Geometry: see drawing. Coordinates: mm, zero at the bounding-box minimum. A direction names the side the tool comes from. Coordinates: 2 decimals unless noted, no trailing zeros. Loops run counter-clockwise (first coordinate to the right, second up) from the corner with the lowest first, then second, coordinate; pieces in that order, holes last. Notation, with made-up numbers: (-17.75, 7.25) -> (10.25, 7.25) arc R16 cw to (10.25, 13.25) -> close; hole circle Ø1 at (29, 40.5). An arc over 180 degrees is marked (long way). Put each result on its own line as item: value. Start each with the question number.
1) Material intervals for L1, parallel to X at y = 45, z = 85; L2, parallel to Z at x = 146.5, y = 40; L3, parallel to Y at x = 135, z = 50 (1 decimal), sorted ascending.
2) Cut plane A-A (x = 267.5). Return the cut outline in (y, z) (1 decimal).
3) Contact query for flat-ended pins moving along their axis: P1, Ø5, axis at x = 65, y = 57.5, coming from the +Z side; P2, Ø4, axis at x = 102.5, y = 37.5, coming from the +Z side; P3, Ø3, axis at x = 94.5, y = 52, coming from the -Z side. Output: stop coordinate, or through.
4) Set-up query: the marked faces 1 and 2. Return all of +Z, -Z, +X, -X, +Y, -Y with unobstructed straight access to the full face (end or side cutting, diameter ignored); none if empty.
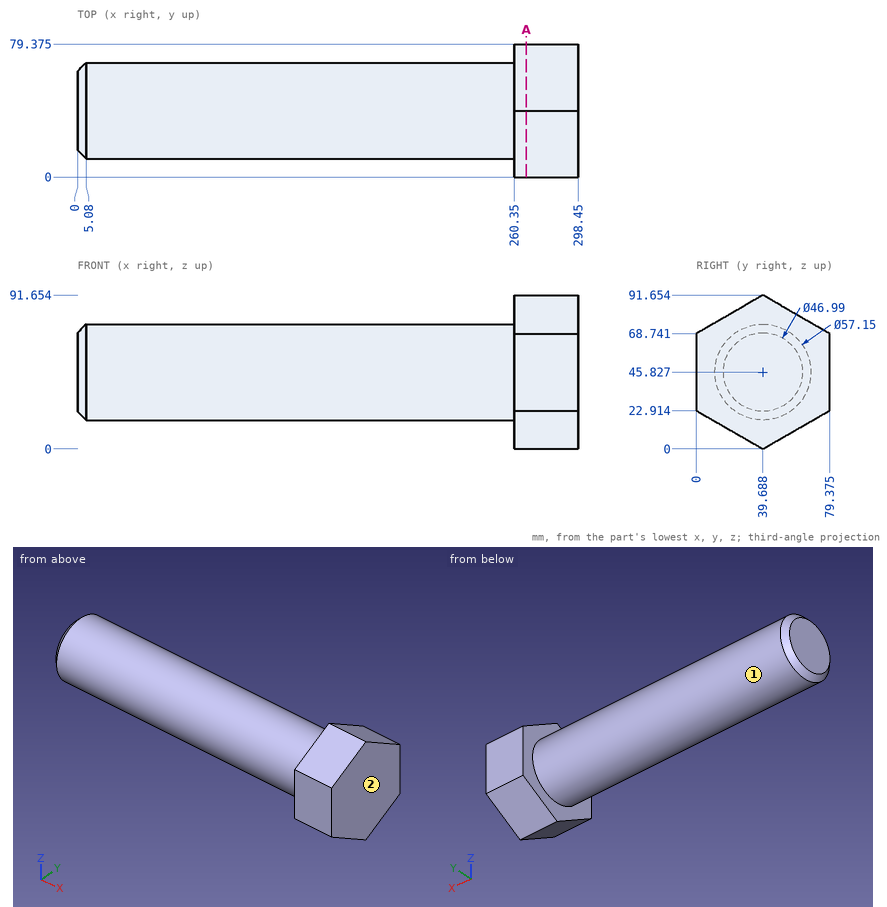
Results found:
1. L1: x = 260.35 to 298.45
1. L2: z = 17.25 to 74.4
1. L3: y = 11.4 to 68
2. outline: (0, 22.9) -> (39.7, 0) -> (79.4, 22.9) -> (79.4, 68.7) -> (39.7, 91.7) -> (0, 68.7) -> close
3. P1: stops at z = 69.95
3. P2: stops at z = 74.4
3. P3: stops at z = 19.38
4. face 1: -X
4. face 2: +Z, -Z, +X, +Y, -Y
